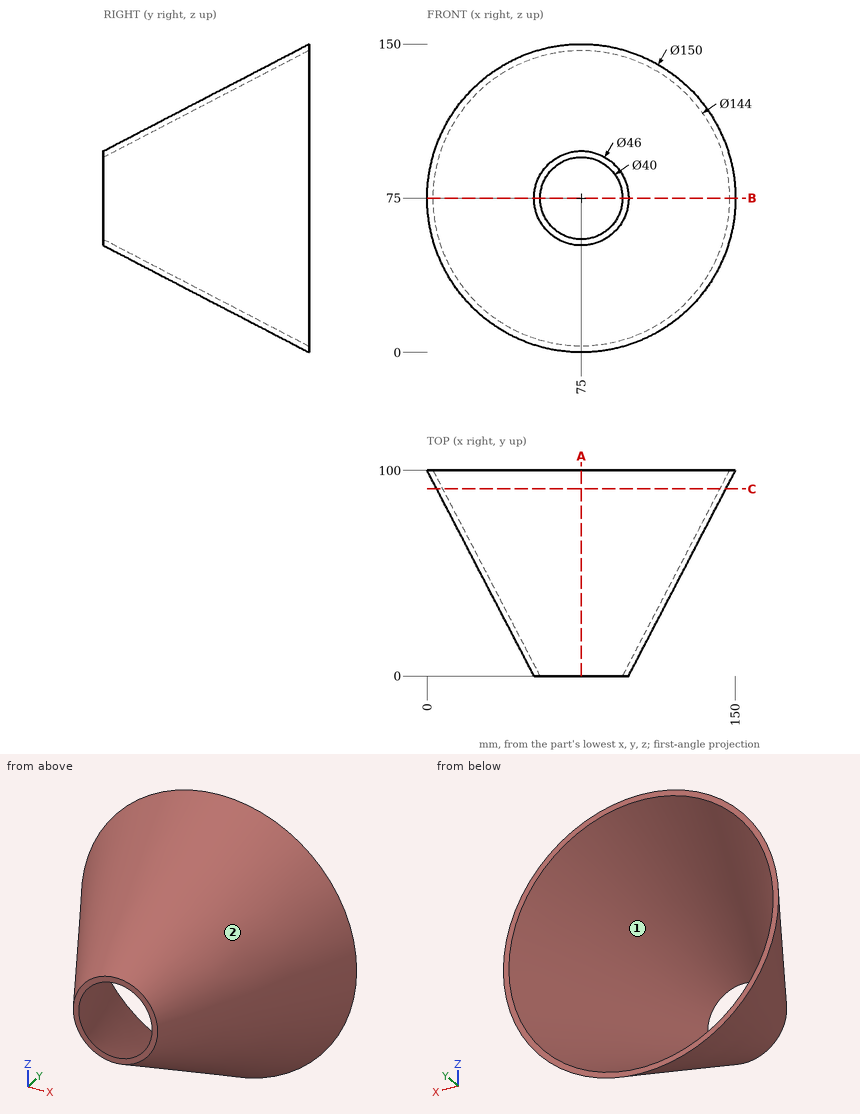
Design review of the part shown in the three views and the two pictorial views. Dimensions are in mm from the part's minimum x, y and z. Coordinates: 2 decimals unless noted, no trailing zeros. Loops run counter-clockwise (first coordinate to the right, second up) from the corner with the lowest first, then second, coordinate; pieces in that order, holes last. Notation, with made-up numbers: M 16,-7 L 48,-7 A21 ccw 48,12 Z; hole C 45,20.25 d8. An arc over 180 degrees is marked long. One line per question, with ' | ' between items.
(1) Draft analysis for pull direction Z (two halves, no side actions). For the marked faces 1 and 2, state which applies: released by +Z, released by -Z, zero draft, split by the parting line, or undercut.
Filled in:
face 1: undercut | face 2: split by the parting line
(2) We need section B-B (z = 75). Give the boundary of the cut face in (x, y).
Filled in:
outline: M 0,100 L 52,0 L 55,0 L 3,100 Z; M 95,0 L 98,0 L 150,100 L 147,100 Z
(3) We need section C-C (y = 91). Give the boundary of the cut face in (x, z), and give its area (3 significant figures).
Filled in:
outline: C 75,75 d140.64; hole C 75,75 d134.64 | area: 1,300 mm^2
(4) We need section A-A (x = 75). Give the boundary of the cut face in (y, z), and give its area (3 significant figures).
Filled in:
outline: M 0,52 L 100,0 L 100,3 L 0,55 Z; M 0,95 L 100,147 L 100,150 L 0,98 Z | area: 600 mm^2
(5) Wall thickness on probe 1 along X at (y, z) = (68.5, 122.5); probe 2 along X at (y, z) = (79, 129.5); probe 3 along Z at (x, y) = (98, 94): over which ranges is each line inside the solid? List them lowest first.
Filled in:
probe 1: x = 40.65 to 46.06, 103.94 to 109.35 | probe 2: x = 41.3 to 47.42, 102.58 to 108.7 | probe 3: z = 6.9 to 10.07, 139.93 to 143.1
(6) For pin 1 Ø6 at (x, z) = (113.5, 134) entering from +Y; pin 2 Ø8 at (x, z) = (38.5, 20.5) entering from +Y; pin 3 Ø4 at (x, z) = (105, 45.5) entering from -Y; pin 4 Ø3 at (x, z) = (111, 47.5) entering from -Y, all flat-tipped, find the tip position at first contact; note any pin that passes through.
Filled in:
pin 1: stops at y = 100 | pin 2: stops at y = 95.37 | pin 3: stops at y = 32.84 | pin 4: stops at y = 40
